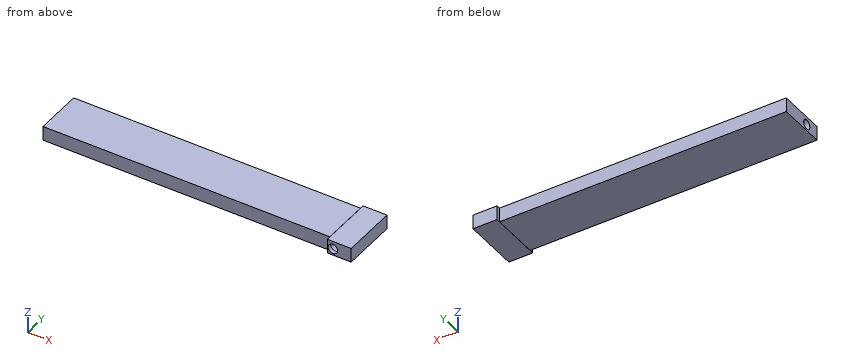
```python
from build123d import *

# Parameters (mm, degrees)
CYLINDER041_R                = 0.6
CYLINDER041_DEPTH            = 40
CYLINDER041_PITCH_ANGLE      = 90
SKETCH004_R                  = 0.6
SWEEP_PLACEMENT_ANGLE        = 180
BOX035_W                     = 3
BOX035_H                     = 7
BOX035_DEPTH                 = 1.8
BOX034_W                     = 1.8
BOX034_H                     = 6
BOX034_DEPTH                 = 36
BOX034_PITCH_ANGLE           = 90
FUSION002018_PLACEMENT_ANGLE = 180


with BuildPart() as cilindro041:
    # Cylinder041 → Cylinder041 (new body)
    with BuildSketch(Plane.XY):
        Circle(CYLINDER041_R)
    extrude(amount=CYLINDER041_DEPTH)


with BuildPart() as cilindro041_1:
    # Cylinder041 pitch: moved
    add(cilindro041.part.rotate(Axis((0, 0, 0), (0, 1, 0)), CYLINDER041_PITCH_ANGLE))


with BuildPart() as cilindro041_2:
    # Cylinder041 placement: moved
    add(cilindro041_1.part.moved(Location((-43, 59, 57))))


with BuildPart() as fusion002020:
    # Sweep: sweep along a path in Sketch002
    with BuildLine(Plane.XY) as sweep_path:
        Line((0, 0), (2.000007, 0))
        ThreePointArc((2.000007, 0), (3.413537, 0.585387), (3.999404, 1.998718))
        Line((3.999404, 1.998718), (3.999404, 3.99963))
    # Sketch004 → Sweep (sweep)
    with BuildSketch(Plane.YZ):
        Circle(SKETCH004_R)
    sweep(path=sweep_path.line, transition=Transition.RIGHT)


with BuildPart() as fusion002020_1:
    # Sweep placement: moved
    add(fusion002020.part.moved(Location((-4.2, 59, 57))).rotate(Axis((-4.2, 59, 57), (1, 0, 0)), SWEEP_PLACEMENT_ANGLE))

    # Fusion002020: union Cilindro041
    add(cilindro041_2.part)


with BuildPart() as cubo035:
    # Box035 → Box035 (new body)
    with BuildSketch(Plane(origin=(-3, -0.5, -1.81873), x_dir=(1, 0, 0), z_dir=(0, 0, 1))):
        with Locations((1.5, 3.5)):
            Rectangle(BOX035_W, BOX035_H)
    extrude(amount=BOX035_DEPTH)


with BuildPart() as cut061:
    # Box034 → Box034 (new body)
    with BuildSketch(Plane.XY):
        with Locations((0.9, 3)):
            Rectangle(BOX034_W, BOX034_H)
    extrude(amount=BOX034_DEPTH)


with BuildPart() as cut061_1:
    # Box034 pitch: moved
    add(cut061.part.rotate(Axis((0, 0, 0), (0, 1, 0)), BOX034_PITCH_ANGLE))


with BuildPart() as cut061_2:
    # Box034 placement: moved
    add(cut061_1.part)

    # Fusion002018: union Cubo035
    add(cubo035.part)


with BuildPart() as cut061_3:
    # Fusion002018 placement: moved
    add(cut061_2.part.moved(Location((-0.9, 63, 58))).rotate(Axis((-0.9, 63, 58), (0, 0, 1)), FUSION002018_PLACEMENT_ANGLE))

    # Cut061: cut Fusion002020
    add(fusion002020_1.part, mode=Mode.SUBTRACT)


with BuildPart() as cut061_4:
    # Cut061 placement: moved
    add(cut061_3.part.moved(Location((0, 0, -11))))


solid = cut061_4.part
```
For this review, take the finished solid that the model builds, in its own axes (mm). Give positions to 0.01 mm unless a question says otherwise; leave off trailing zeros. Order: outer loops, then holes, each group sorted by start corner. A loop starts at its lowest first (then second) coordinate and runs counter-clockwise, first axis right, second up.
1) Insertion check: pin 1 (0.9 mm diameter, centred on x = -21.5, z = 46, fed in from -Y); pin 2 (4 mm diameter, centred on x = -21.5, y = 59, fed in from -Z); pin 3 (3.5 mm diameter, centred on x = 0, y = 58.5, fed in from +Z). Each pin has a flat end and moves straight along its axis. Give the tip position at first contact, or say it passes through.
2) Wall thickness on line 1 (Z direction, x = -3.25, y = 59); line 2 (Y direction, x = -11.5, z = 46); line 3 (X direction, y = 63.25, z = 46.65): over which ranges is each line inside the solid? List them lowest first.
3) Take a section at A-A (x = -33.5). Give the boundary of the cut face in (y, z).
Derived:
1. pin 1: stops at y = 57
1. pin 2: stops at z = 45.2
1. pin 3: stops at z = 47
2. line 1: z = 45.2 to 45.4, 46.6 to 47
2. line 2: y = 57 to 58.4, 59.6 to 63
2. line 3: x = -0.9 to 2.1
3. outline: (57, 45.2) - (63, 45.2) - (63, 47) - (57, 47) - close; hole circle Ø1.2 at (59, 46)
